```python
from build123d import *

# Parameters (mm, degrees)
SKETCH_1_W          = 110
SKETCH_1_H          = 120
EXTRUDE_1_DEPTH     = 130
SKETCH_3_W          = 75.6
SKETCH_3_H          = 120
CUT_EXTRUDE_1_DEPTH = 130
EXTRUDE_2_DEPTH     = 5
EXTRUDE_3_DEPTH     = 110
FILLET_START        = -8.112141349
FILLET_2_DEPTH      = 28.712141349
FILLET_START_2      = -55
FILLET_2_2_DEPTH    = 110
FILLET_3_R          = 60
FILLET_4_R          = 5
SKETCH_6_R          = 49.5
CUT_EXTRUDE_2_DEPTH = 27.7
SKETCH_7_R          = 29.5
CUT_EXTRUDE_5_DEPTH = 177.552797006
SKETCH_8_R          = 2.5
SKETCH_8_R_2        = 2
CUT_EXTRUDE_6_DEPTH = 10


with BuildPart() as part:
    # 草图1 → 凸台-拉伸1 (new body)
    with BuildSketch(Plane(origin=(0, 0, 0), x_dir=(1, 0, 0), z_dir=(0, 1, 0))):
        Rectangle(SKETCH_1_W, SKETCH_1_H)
    extrude(amount=EXTRUDE_1_DEPTH)

    # 草图3 → 切除-拉伸1 (cut)
    with BuildSketch(Plane.XY.offset(60)):
        with Locations((-17.2, 70)):
            Rectangle(SKETCH_3_W, SKETCH_3_H)
    extrude(amount=-CUT_EXTRUDE_1_DEPTH, mode=Mode.SUBTRACT)

    # 草图4 → 凸台-拉伸2 (add)
    with BuildSketch(Plane.XY.offset(60)):
        with BuildLine():
            Line((20.6, 130), (15.6, 130))
            add(Edge.make_bspline(
                [(-55, 10), (-2.665013162, 59.248795935), (15.6, 130)],
                knots=[0, 0, 0, 1, 1, 1], degree=2))
            Line((-55, 10), (20.6, 10))
            Line((20.6, 10), (20.6, 130))
        make_face()
    extrude_2 = extrude(amount=-EXTRUDE_2_DEPTH)

    # 镜向1: 凸台-拉伸2 across plane
    add(extrude_2.mirror(Plane.XY))

    # 草图5 → 凸台-拉伸3 (add)
    with BuildSketch(Plane(origin=(0, 0, 55), x_dir=(-1, 0, 0), z_dir=(0, 0, -1))):
        with BuildLine():
            Line((-20.6, 130), (-20.6, 125))
            Line((-20.6, 125), (-14.2592003, 125))
            add(Edge.make_bspline(
                [(-14.259200299, 125), (-14.95110103, 127.486430307), (-15.600000021, 130.000000082)],
                knots=[0.964473117, 0.964473117, 0.964473117, 1, 1, 1], degree=2))
            Line((-15.600000021, 130.000000082), (-20.6, 130))
        make_face()
    extrude(amount=EXTRUDE_3_DEPTH)

    # 圆角2: read off the stored shape, not the designer's step
    # 圆角2 outline → 圆角2 (add)
    with BuildSketch(Plane.YZ.offset(FILLET_START)):
        with BuildLine():
            Line((125, 55), (70, 55))
            ThreePointArc((70, 55), (108.890872965, 38.890872965), (125, 0))
            Line((125, 0), (125, 55))
        make_face()
        with BuildLine():
            Line((125, -55), (125, 0))
            ThreePointArc((125, 0), (108.890872965, -38.890872965), (70, -55))
            Line((70, -55), (125, -55))
        make_face()
    extrude(amount=FILLET_2_DEPTH)

    # Fillet 2 2 outline → Fillet 2 2 (cut)
    with BuildSketch(Plane.XY.offset(FILLET_START_2)):
        with BuildLine():
            add(Edge.make_bspline(
                [(14.259200299, 125), (6.078935587, 95.603213424), (-8.112141272, 69.999999958)],
                knots=[0.035526883, 0.035526883, 0.035526883, 0.455557239, 0.455557239, 0.455557239], degree=2))
            Line((14.259200299, 125), (-8.112141349, 125))
            Line((-8.112141349, 125), (-8.112141272, 69.999999958))
        make_face()
    extrude(amount=FILLET_2_2_DEPTH, mode=Mode.SUBTRACT)

    # 圆角3
    # the kernel refuses this fillet: 60 mm, written as the material it takes off along each edge
    with BuildSketch(Plane(origin=(205, 130, 60), x_dir=(0, -1, 0), z_dir=(-1, 0, 0)), Plane(origin=(205, 130, -60), x_dir=(0, 0, 1), z_dir=(-1, 0, 0))) as fillet_3_piece_1:
        with BuildLine():
            CenterArc((FILLET_3_R, -FILLET_3_R), FILLET_3_R, 90, 90)
            Line((0, -FILLET_3_R), (0, 0))
            Line((0, 0), (FILLET_3_R, 0))
        make_face()
    extrude(amount=339.4, mode=Mode.SUBTRACT)

    # 圆角4
    fillet_4_edges = [part.edges().sort_by_distance(p)[0] for p in [
        (-55, 5, 60),
        (-55, 5, -60),
    ]]
    fillet(fillet_4_edges, radius=FILLET_4_R)

    # 草图6 → 切除-拉伸2 (cut)
    with BuildSketch(Plane.ZY.offset(-20.6)):
        with Locations(Location((0, 72.500997163, 0), (0, 0, 270))):
            Circle(SKETCH_6_R)
    extrude(amount=-CUT_EXTRUDE_2_DEPTH, mode=Mode.SUBTRACT)

    # 草图7 → 切除-拉伸5 (cut, through all)
    with BuildSketch(Plane.ZY.offset(-48.3)):
        with Locations(Location((0, 72.500997163, 0), (0, 0, 270))):
            Circle(SKETCH_7_R)
    extrude(amount=-CUT_EXTRUDE_5_DEPTH, mode=Mode.SUBTRACT)

    # 草图8 → 切除-拉伸6 (cut)
    with BuildSketch(Plane.XZ):
        with Locations(Location((0, 0, 0), (0, 0, 270))):
            Circle(SKETCH_8_R)
        with Locations(Location((0, 17.25, 0), (0, 0, 270))):
            Circle(SKETCH_8_R_2)
        with Locations(Location((0, -17.25, 0), (0, 0, 270))):
            Circle(SKETCH_8_R_2)
    extrude(amount=-CUT_EXTRUDE_6_DEPTH, mode=Mode.SUBTRACT)


solid = part.part
```
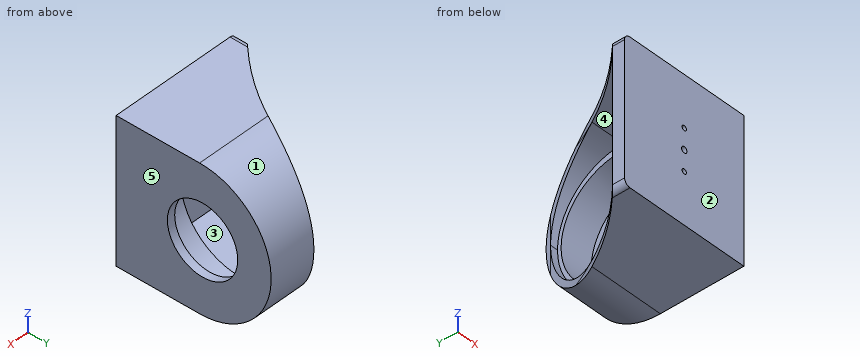
The model under review builds one solid part; all positions refer to its coordinate system, in mm. Face numbers are marked on the shaded views. A direction names the side the tool comes from. Coordinates: 2 decimals unless noted, no trailing zeros. Order: outer loops, then holes, each group sorted by start corner. A loop starts at its lowest first (then second) coordinate and runs counter-clockwise, first axis right, second up. Notation, with made-up numbers: M -39.5,-36 L 18.5,-36 A25 ccw 18.5,-24 Z; hole C 53,36 d10. An arc over 180 degrees is marked long. One line per question, with ' | ' between items.
(1) Machinability: for the marked faces 4 and 5, which of the approach directions +Z, -Z, +X, -X, +Y, -Y give a long, thin tool a straight path to every point of the face, cutting with its end or side? Answer none if there is none.
Geometry results:
face 4: -X | face 5: +Z, -Z, +X, +Y, -Y
(2) For probe 1 along X at (y, z) = (3, 0); probe 2 along X at (y, z) = (4, -17); probe 3 along Z at (x, y) = (1.5, 48), list the stretches that pass through material, from the lowest coordinate up. Write a range as from..to.
Geometry results:
probe 1: x = -55..-2.5, 2.5..55 | probe 2: x = -55..-1.98, 1.98..55 | probe 3: z = -60..-55, 55..60
(3) Add section A-A, the plane x = 44. Write out the cut boundary in (y, z), then the cut area to 3 significant figures.
Geometry results:
outline: M 0,-60 L 70,-60 A60 ccw 70,60 L 0,60 Z; hole C 72.5,0 d99 | area: 6,360 mm²
(4) Insertion check: pin 1 (6.5 mm diameter, centred on x = 0, z = 17.25, fed in from -Y); pin 2 (8 mm diameter, centred on x = 2, y = 83.5, fed in from +Z); pin 3 (4 mm diameter, centred on y = 23, z = -13, fed in from -X); pin 4 (6.5 mm diameter, centred on x = 0, z = -17.25, fed in from +Y). Each pin has a flat end and moves straight along its axis. Give the tip position at first contact, or say it passes through.
Geometry results:
pin 1: stops at y = 0 | pin 2: stops at z = 59.24 | pin 3: stops at x = 20.6 | pin 4: stops at y = 10
(5) Add section B-B, the plane z = 17.25. State how many separate pieces and enclosed holes the cut face has, then the cut area to 3 significant figures.
Geometry results:
separate pieces: 3 | enclosed holes: 0 | area: 2,240 mm²
(6) The part is to be moulded in two halves that separate along Y. For the marked faces 1, 2 and 3, say which applies: +Y half, -Y half, draft (parallel to the pull), parting line (faces both ways), or undercut.
Geometry results:
face 1: +Y half | face 2: -Y half | face 3: undercut
